```python
from build123d import *

# Parameters (mm, degrees)
PAD006_DEPTH    = 5
SKETCH040_R     = 3.2
POCKET034_DEPTH = 5
SKETCH041_W     = 163
SKETCH041_H     = 205
PAD007_DEPTH    = 5
SKETCH042_W     = 205
SKETCH042_H     = 176.4
PAD008_DEPTH    = 5
SKETCH043_W     = 149
SKETCH043_H     = 199
POCKET035_DEPTH = 5
SKETCH049_R     = 2.2
POCKET040_DEPTH = 5


with BuildPart() as part:
    # Sketch039 → Pad006 (new body)
    with BuildSketch(Plane.XY):
        with BuildLine():
            Line((-100, 110), (100, 110))
            ThreePointArc((110, 100), (107.071068, 107.071068), (100, 110))
            Line((110, 100), (110, -100))
            ThreePointArc((100, -110), (107.071068, -107.071068), (110, -100))
            Line((100, -110), (-100, -110))
            ThreePointArc((-110, -100), (-107.071068, -107.071068), (-100, -110))
            Line((-110, -100), (-110, 100))
            ThreePointArc((-100, 110), (-107.071068, 107.071068), (-110, 100))
        make_face()
    extrude(amount=PAD006_DEPTH)

    # Sketch040 (on Face10 of Pad006) → Pocket034 (cut)
    with BuildSketch(Plane.XY.offset(5)):
        with Locations((-94.5, 99.1)):
            Circle(SKETCH040_R)
        with Locations((94.5, 99.1)):
            Circle(SKETCH040_R)
        with Locations((94.5, -99.1)):
            Circle(SKETCH040_R)
        with Locations((-94.5, -99.1)):
            Circle(SKETCH040_R)
    extrude(amount=-POCKET034_DEPTH, mode=Mode.SUBTRACT)

    # Sketch041 (on Face4 of Pocket034) → Pad007 (join)
    with BuildSketch(Plane(origin=(0, 0, 0), x_dir=(1, 0, 0), z_dir=(0, 0, -1))):
        Rectangle(SKETCH041_W, SKETCH041_H)
    extrude(amount=PAD007_DEPTH)

    # Sketch042 (on Face4 of Pocket034) → Pad008 (join)
    with BuildSketch(Plane(origin=(0, 0, 0), x_dir=(1, 0, 0), z_dir=(0, 0, -1))):
        Rectangle(SKETCH042_W, SKETCH042_H)
    extrude(amount=PAD008_DEPTH)

    # Sketch043 (on Face31 of Pad008) → Pocket035 (cut)
    with BuildSketch(Plane(origin=(0, 0, -5), x_dir=(1, 0, 0), z_dir=(0, 0, -1))):
        Rectangle(SKETCH043_W, SKETCH043_H)
    extrude(amount=-POCKET035_DEPTH, mode=Mode.SUBTRACT)

    # Sketch049 → Pocket040 (cut)
    with BuildSketch(Plane.XY):
        with Locations((-40, 81.965103)):
            Circle(SKETCH049_R)
        with Locations((40, 81.965103)):
            Circle(SKETCH049_R)
        with Locations((40, 1.965103)):
            Circle(SKETCH049_R)
        with Locations((-40, 1.965103)):
            Circle(SKETCH049_R)
    extrude(amount=POCKET040_DEPTH, mode=Mode.SUBTRACT)


with BuildPart() as part_1:
    # Body004 placement: moved
    add(part.part.moved(Location((0, 0, 229.4))))


solid = part_1.part
```
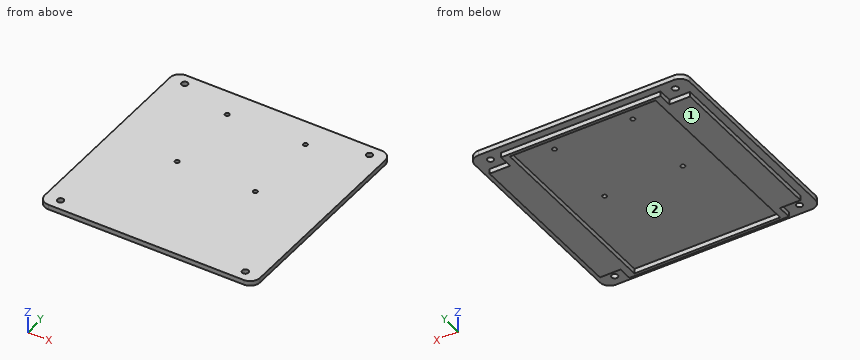
Here's how the part is built. I have some questions about the finished solid (model axes, mm). Face numbers are marked on the shaded views. Round coordinates to 2 decimals unless told otherwise and drop trailing zeros. Write each loop counter-clockwise with the first axis right and the second up, starting at its lowest first coordinate (ties: lowest second). Pieces come first, ordered by that corner, then holes. Notation, with made-up numbers: M 37.5,-5.75 L 52.5,-5.75 A7 cw 52.5,5.25 Z; hole C 1,32 d7. An arc over 180 degrees is marked long. Answer as CSV lines item,"result". Start each with the question number.
1. Suppose I cut it at A-A on x = -94.5. Write out the boundary of the cut face in (y, z).
2. Suppose I cut it at D-D on x = -64.5. Write out the boundary of the cut face in (y, z), then the cut area to 3 significant figures.
3. Suppose I cut it at B-B on z = 226.5. Write out the boundary of the cut face in (x, y).
4. Thinking about a two-plate mould opening in Y: for the marked faces 1 and 2, which applies, released by +Y, released by -Y, zero draft, split by the parting line, or undercut?
5. I'm going to push flat-ended pins straight in: pin 1 Ø4 at (y, z) = (-42, 226.5) entering from +X; pin 2 Ø2.5 at (x, z) = (-94.5, 226) entering from -Y; pin 3 Ø1.5 at (x, z) = (90, 227) entering from +Y. Where does each tip first touch, or does it pass through?
6. I need wall thicknesses on probe 1 along Y at (x, z) = (-40, 232.45); probe 2 along X at (y, z) = (19, 226.5); probe 3 along X at (y, z) = (97.5, 232). Which ranges of each line are inside material? Lowest first, please.
7. Suppose I cut it at C-C on y = -26.5. Write out the boundary of the cut face in (x, z), then the cut area to 3 significant figures.
Check result:
1,outline,"M -110,229.4 L -102.3,229.4 L -102.3,234.4 L -110,234.4 Z; M -95.9,229.4 L -88.2,229.4 L -88.2,224.4 L 88.2,224.4 L 88.2,229.4 L 95.9,229.4 L 95.9,234.4 L -95.9,234.4 Z; M 102.3,229.4 L 110,229.4 L 110,234.4 L 102.3,234.4 Z"
2,outline,"M -110,229.4 L -102.5,229.4 L -102.5,224.4 L -99.5,224.4 L -99.5,229.4 L 99.5,229.4 L 99.5,224.4 L 102.5,224.4 L 102.5,229.4 L 110,229.4 L 110,234.4 L -110,234.4 Z"
2,area,"1,130 mm2"
3,outline,"M -102.5,-88.2 L -81.5,-88.2 L -81.5,-102.5 L 81.5,-102.5 L 81.5,-88.2 L 102.5,-88.2 L 102.5,88.2 L 81.5,88.2 L 81.5,102.5 L -81.5,102.5 L -81.5,88.2 L -102.5,88.2 Z; hole M -74.5,-99.5 L 74.5,-99.5 L 74.5,99.5 L -74.5,99.5 Z"
4,face 1,"zero draft"
4,face 2,"undercut"
5,pin 1,"stops at x = 102.5"
5,pin 2,"stops at y = -88.2"
5,pin 3,"stops at y = 88.2"
6,probe 1,"y = -110 to -0.23, 4.17 to 79.77, 84.17 to 110"
6,probe 2,"x = -102.5 to -74.5, 74.5 to 102.5"
6,probe 3,"x = -110 to -97.27, -91.73 to 91.73, 97.27 to 110"
7,outline,"M -110,229.4 L -102.5,229.4 L -102.5,224.4 L -74.5,224.4 L -74.5,229.4 L 74.5,229.4 L 74.5,224.4 L 102.5,224.4 L 102.5,229.4 L 110,229.4 L 110,234.4 L -110,234.4 Z"
7,area,"1,380 mm2"
